Verification items for the finished model (mm, model axes). A direction names the side the tool comes from. Round coordinates to 2 decimals unless told otherwise and drop trailing zeros. Loops run counter-clockwise (first coordinate to the right, second up) from the corner with the lowest first, then second, coordinate; pieces in that order, holes last. Notation, with made-up numbers: (-12.5, 44) -> (22.5, 44) arc R26 ccw to (22.5, 80) -> close; hole circle Ø10 at (24, 68.5). An arc over 180 degrees is marked (long way). Write item = value, one per line.
```python
from build123d import *

# Parameters (mm, degrees)
SKETCH1_R           = 1.5
BOSS_EXTRUDE1_DEPTH = 5
SKETCH2_R           = 1.5
BOSS_EXTRUDE2_DEPTH = 5
SPLIT6_START        = -34.5
SPLIT6_DEPTH        = 30
SKETCH24_R          = 2.5
CUT_EXTRUDE3_DEPTH  = 149.21791213


# Read off the part's stored shape, not the designer's step: Split6
with BuildPart() as part:
    # Sketch1 → Boss-Extrude1 (new body)
    with BuildSketch(Plane.XY):
        with BuildLine():
            Line((-20, 10), (20, 10))
            Line((20, 10), (20, -10))
            Line((20, -10), (-20, -10))
            ThreePointArc((-20, -10), (-30, 0), (-20, 10))
        make_face()
        with Locations((-20, 0)):
            Circle(SKETCH1_R, mode=Mode.SUBTRACT)
        with Locations((-20, -7)):
            Circle(SKETCH1_R, mode=Mode.SUBTRACT)
        with Locations((-27, 0)):
            Circle(SKETCH1_R, mode=Mode.SUBTRACT)
        with Locations((-20, 7)):
            Circle(SKETCH1_R, mode=Mode.SUBTRACT)
        with Locations((-13, 0)):
            Circle(SKETCH1_R, mode=Mode.SUBTRACT)
    extrude(amount=BOSS_EXTRUDE1_DEPTH)



with BuildPart() as body_2:
    # Sketch2 → Boss-Extrude2 (new body)
    with BuildSketch(Plane(origin=(0, 0, -39), x_dir=(-1, 0, 0), z_dir=(0, 0, -1))):
        with BuildLine():
            Line((-20, 10), (20, 10))
            ThreePointArc((20, 10), (30, 0), (20, -10))
            Line((20, -10), (-20, -10))
            Line((-20, -10), (-20, 10))
        make_face()
        with Locations(Location((20, 0, 0), (0, 0, 180))):
            Circle(SKETCH2_R, mode=Mode.SUBTRACT)
        with Locations(Location((13, 0, 0), (0, 0, 180))):
            Circle(SKETCH2_R, mode=Mode.SUBTRACT)
        with Locations(Location((20, 7, 0), (0, 0, 180))):
            Circle(SKETCH2_R, mode=Mode.SUBTRACT)
        with Locations(Location((27, 0, 0), (0, 0, 180))):
            Circle(SKETCH2_R, mode=Mode.SUBTRACT)
        with Locations(Location((20, -7, 0), (0, 0, 180))):
            Circle(SKETCH2_R, mode=Mode.SUBTRACT)
    extrude(amount=BOSS_EXTRUDE2_DEPTH)

    # Sketch12 → section 1 of loft1
    with BuildSketch(Plane(origin=(65, 0, 0), x_dir=(0, 0, -1), z_dir=(1, 0, 0)), mode=Mode.PRIVATE) as loft1_s1:
        with BuildLine():
            Line((4.5, 50), (34.5, 50))
            Line((34.5, 50), (34.5, 20))
            Line((34.5, 20), (4.5, 20))
            Line((4.5, 20), (4.5, 50))
        make_face()
    # loft from a face of the part (loft1)
    loft([body_2.faces().sort_by_distance((20, 0, -41.5))[0], loft1_s1.sketch])


with BuildPart() as part_1:
    add(part.part)

    add(body_2.part)  # loft2 joins it to this body
    # loft from a face of the part (loft2)
    loft([part_1.faces().sort_by_distance((20, 0, 2.5))[0], part_1.faces().sort_by_distance((65, 35, -19.5))[0]])

    # Sketch18 → section 1 of loft3
    with BuildSketch(Plane(origin=(140, 0, 0), x_dir=(0, 0, -1), z_dir=(1, 0, 0)), mode=Mode.PRIVATE) as loft3_s1:
        with BuildLine():
            Line((4.5, 82), (34.5, 82))
            Line((34.5, 82), (34.5, 52))
            Line((34.5, 52), (4.5, 52))
            Line((4.5, 52), (4.5, 82))
        make_face()
    # loft from a face of the part (loft3)
    loft([part_1.faces().sort_by_distance((65, 35, -19.5))[0], loft3_s1.sketch])

    # Split6 outline → Split6 (cut)
    with BuildSketch(Plane.XY.offset(SPLIT6_START)):
        with BuildLine():
            ThreePointArc((106.079345998, 67.527187626), (124.183572198, 60.251657472), (116.908042043, 42.147431272))
            Line((116.908042043, 42.147431272), (140, 52))
            Line((140, 52), (140, 82))
            Line((140, 82), (106.079345998, 67.527187626))
        make_face()
    extrude(amount=SPLIT6_DEPTH, mode=Mode.SUBTRACT)

    # Sketch24 → Cut-Extrude3 (cut, through all)
    with BuildSketch(Plane.XY.offset(-4.5)):
        with Locations((119.739276472, 59.632240301)):
            Circle(SKETCH24_R)
    extrude(amount=-CUT_EXTRUDE3_DEPTH, mode=Mode.SUBTRACT)


solid = part_1.part
```
(1) Go/stop test with flat-tipped pins: pin 1 Ø2 at (x, y) = (108, 38.5) entering from -Z; pin 2 Ø8 at (x, z) = (52, -18.5) entering from -Y; pin 3 Ø10 at (x, z) = (39.5, -30.5) entering from -Y. Record where each tip stops, or that it passes through.
Filled sheet:
pin_1 = -34.5
pin_2 = 8.67
pin_3 = -0.33
(2) Sectioned sample at A-A, the plane x = -16.5. Record the cut outline in (y, z).
Filled sheet:
outline = (-10, -44) -> (10, -44) -> (10, -39) -> (-10, -39) -> close; (-10, 0) -> (10, 0) -> (10, 5) -> (-10, 5) -> close
(3) Draft check along Y on faces 4 (the face through (120.893, 57.414, -19.29)), 5 (the face through (-14.5, -0.07, -41.46)), 6 (the face through (91.32, 31.23, -19.29)), 7 (the face through (-30, 0, -41)). Enter one of: released by +Y, released by -Y, zero draft, split by the parting line, or undercut.
Filled sheet:
face_4 = undercut
face_5 = undercut
face_6 = released by -Y
face_7 = split by the parting line
(4) Sectioned sample at B-B, the plane y = 0. Count the separate pieces of the cut face and the enclosed holes in it, and give its area (3 significant figures).
Filled sheet:
separate_pieces = 8
enclosed_holes = 0
area = 685 mm2
(5) Material ranges on probe 1 along Y at (x, z) = (-20, 4.05); probe 2 along Z at (x, y) = (-12.5, 5.5); probe 3 along Z at (x, y) = (90, 46.5), recorded low to high. Write a range as from..to.
Filled sheet:
probe_1 = -10..-8.5, -5.5..-1.5, 1.5..5.5, 8.5..10
probe_2 = -44..-39, 0..5
probe_3 = -34.5..-4.5
(6) Set-up check for faces 1 (the face through (-21.5, 6.93, -41.46)), 2 (the face through (0, 10, -41)), 3 (the face through (-5, 0, 0)): record each of +Z, -Z, +X, -X, +Y, -Y from which the full face is reachable in a straight line by a thin tool's end or side.
Filled sheet:
face_1 = +Z, -Z
face_2 = +Z, -Z, -X, +Y
face_3 = -X, +Y, -Y
